Geometry: final body of the model. Coordinates: model frame, mm. Face numbers are marked on the shaded views. A direction names the side the tool comes from. Coordinates: 2 decimals unless noted, no trailing zeros. Order: outer loops, then holes, each group sorted by start corner. A loop starts at its lowest first (then second) coordinate and runs counter-clockwise, first axis right, second up. Notation, with made-up numbers: (49.5, 84.5) -> (106.5, 84.5) arc R11 ccw to (106.5, 99.5) -> close; hole circle Ø1 at (60.25, -39.5). An arc over 180 degrees is marked (long way). Answer in a Markdown table with one row per item. Add a question column.
1) Set-up query: the marked faces 1 and 2. Return all of +Z, -Z, +X, -X, +Y, -Y with unobstructed straight access to the full face (end or side cutting, diameter ignored); none if empty.
2) Section query A-A on y = 1.25. Return the cut outline in (x, z), then the cut area to 3 significant figures.
3) Ray query, line 1 (Y direction, x = -1.75, z = 36.5); line 2 (X direction, y = 3, z = 40.5); line 3 (Z direction, x = -4, y = 6). Return the intervals inside material, ascending. Write a range as from..to.
4) Contact query for flat-ended pins moving along their axis: P1, Ø2, axis at x = 1, z = 43.5, coming from the -Y side; P2, Ø2, axis at x = 1, z = 36, coming from the +Y side. Output: stop coordinate, or through.
5) Section query B-B on y = 8.5. Return the cut outline in (x, z).
```python
from build123d import *

# Parameters (mm, degrees)
SKETCH1_R           = 9.1
BOSS_EXTRUDE5_DEPTH = 2
SKETCH4_R           = 5
BOSS_EXTRUDE6_DEPTH = 8
CUT_EXTRUDE2_DEPTH  = 0.5
FILLET1_R           = 0.5


with BuildPart() as part:
    # Sketch1 → Boss-Extrude5 (new body)
    with BuildSketch(Plane(origin=(0, 0, 0), x_dir=(1, 0, 0), z_dir=(0, 1, 0))):
        with Locations(Location((-5.408676197, -40.3067379, 0), (0, 0, 270))):
            Circle(SKETCH1_R)
    extrude(amount=BOSS_EXTRUDE5_DEPTH)

    # Sketch4 → Boss-Extrude6 (add)
    with BuildSketch(Plane(origin=(0, 2, 0), x_dir=(1, 0, 0), z_dir=(0, 1, 0))):
        with Locations(Location((-5.408676197, -40.3067379, 0), (0, 0, 270))):
            Circle(SKETCH4_R)
    extrude(amount=BOSS_EXTRUDE6_DEPTH)

    # Sketch5 → Cut-Extrude2 (cut)
    with BuildSketch(Plane.XZ):
        Polygon((-6.443159021, 44.805369713), (-4.485226328, 44.805369713), (-4.485226328, 35.805369713), (-5.639072482, 35.805369713), (-5.639072482, 43.766908174), (-7.023687867, 43.766908174), align=None)
    extrude(amount=-CUT_EXTRUDE2_DEPTH, mode=Mode.SUBTRACT)

    # Fillet1
    fillet1_edges = [part.edges().sort_by_distance(p)[0] for p in [
        (-5.408676197, 0, 31.2067379),
        (-5.408676197, 2, 31.2067379),
    ]]
    fillet(fillet1_edges, radius=FILLET1_R)


solid = part.part
```
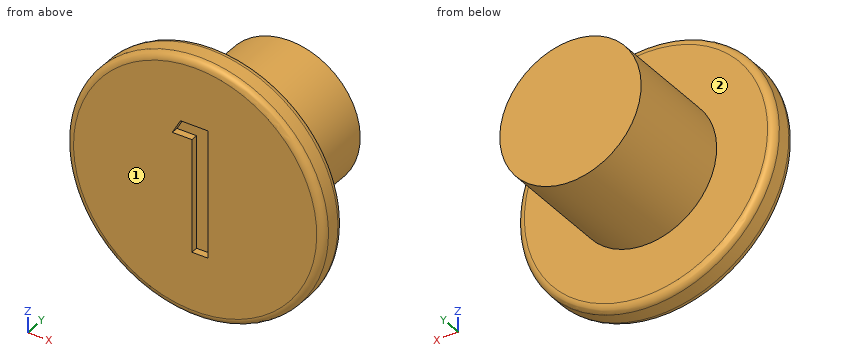
Result:
| question | item | result |
|---|---|---|
| 1 | face 1 | +Z, -Z, +X, -X, -Y |
| 1 | face 2 | +Y |
| 2 | outline | circle Ø18.2 at (-5.41, 40.31) |
| 2 | area | 260 mm2 |
| 3 | line 1 | 0..2 |
| 3 | line 2 | -10.4..-0.41 |
| 3 | line 3 | 35.51..45.1 |
| 4 | P1 | y = 0 |
| 4 | P2 | y = 2 |
| 5 | outline | circle Ø10 at (-5.41, 40.31) |
